Can you work these out from the model? Positions are in its coordinate system, mm. A direction names the side the tool comes from. Coordinates: 2 decimals unless noted, no trailing zeros. Order: outer loops, then holes, each group sorted by start corner. A loop starts at its lowest first (then second) coordinate and runs counter-clockwise, first axis right, second up. Notation, with made-up numbers: M -9.5,-7 L 36.5,-7 A26 ccw 36.5,29 Z; hole C -8.75,13 d3. An arc over 180 degrees is marked long. Answer as a JSON object with one key per item and string values.
from build123d import *

# Parameters (mm, degrees)
SKETCH1_W             = 28.575
SKETCH1_H             = 81.28
BOSS_EXTRUDE1_DEPTH   = 4.7625
SKETCH2_W             = 19.05
SKETCH2_H             = 25.4
CUT_EXTRUDE1_DEPTH    = 44.340785209
FILLET1_R             = 3.302
F_4_40_TAPPED_HOLE1_D = 2.2606


with BuildPart() as part:
    # Sketch1 → Boss-Extrude1 (new body)
    with BuildSketch(Plane.XY):
        Rectangle(SKETCH1_W, SKETCH1_H)
    extrude(amount=BOSS_EXTRUDE1_DEPTH)

    # Sketch2 → Cut-Extrude1 (cut, through all)
    with BuildSketch(Plane.XY.offset(4.7625)):
        with Locations((0, 17.78)):
            Rectangle(SKETCH2_W, SKETCH2_H)
        with Locations((0, -17.78)):
            Rectangle(SKETCH2_W, SKETCH2_H)
    extrude(amount=-CUT_EXTRUDE1_DEPTH, mode=Mode.SUBTRACT)

    # Fillet1
    fillet1_edges = [part.edges().sort_by_distance(p)[0] for p in [
        (9.525, 30.48, 2.38125),
        (9.525, 5.08, 2.38125),
        (-9.525, 5.08, 2.38125),
        (-9.525, 30.48, 2.38125),
        (-9.525, -30.48, 2.38125),
        (-9.525, -5.08, 2.38125),
        (9.525, -5.08, 2.38125),
        (9.525, -30.48, 2.38125),
    ]]
    fillet(fillet1_edges, radius=FILLET1_R)

    # #4-40 Tapped Hole1 (through all)
    with Locations(Plane(origin=(14.2875, 0, 0), x_dir=(0, 0, -1), z_dir=(1, 0, 0))):
        with Locations((-2.38125, 35.56), (-2.38125, 0), (-2.38125, -35.56)):
            Hole(F_4_40_TAPPED_HOLE1_D / 2)


solid = part.part
Item 1: I want a section at A-A, the plane x = -5.5. Write out the boundary of the cut face in (y, z).
Answers follow:
{"outline": "M -40.64,0 L -30.48,0 L -30.48,4.76 L -40.64,4.76 Z; M -5.08,0 L 5.08,0 L 5.08,4.76 L -5.08,4.76 Z; M 30.48,0 L 40.64,0 L 40.64,4.76 L 30.48,4.76 Z; hole C -35.56,2.38 d2.26; hole C 0,2.38 d2.26; hole C 35.56,2.38 d2.26"}
Item 2: Please list where these lines run through material, in increasing order: line 1 (Y direction, x = -6.5, z = 1); line 2 (X direction, y = -9, z = 0.4) (1 decimal); line 3 (Y direction, x = -6.25, z = 2.7).
Answers follow:
{"line 1": "y = -40.64 to -30.47, -5.09 to 5.09, 30.47 to 40.64", "line 2": "x = -14.3 to -9.5, 9.5 to 14.3", "line 3": "y = -40.64 to -36.64, -34.48 to -30.48, -5.08 to -1.08, 1.08 to 5.08, 30.48 to 34.48, 36.64 to 40.64"}
Item 3: I want a section at C-C, the plane y = -20. Write out the boundary of the cut face in (x, z) (1 decimal), plus the area to 3 significant figures.
Answers follow:
{"outline": "M -14.3,0 L -9.5,0 L -9.5,4.8 L -14.3,4.8 Z; M 9.5,0 L 14.3,0 L 14.3,4.8 L 9.5,4.8 Z", "area": "45.4 mm^2"}
Item 4: Which directions (+Z, -Z, +X, -X, +Y, -Y) give clear straight access to the entire face, cutting with the end or side of a thin tool? Please do faces 4 (the flat face through (0, 40.64, 2)), 5 (the cylindrical face through (-8.53, 29.54, 2.35)).
Answers follow:
{"face 4": "+Z, -Z, +X, -X, +Y", "face 5": "+Z, -Z"}
Item 5: I want a section at B-B, the plane y = 35.56. Write out the boundary of the cut face in (x, z), plus the area to 3 significant figures.
Answers follow:
{"outline": "M -14.29,0 L 14.29,0 L 14.29,1.25 L -14.29,1.25 Z; M -14.29,3.51 L 14.29,3.51 L 14.29,4.76 L -14.29,4.76 Z", "area": "71.5 mm^2"}
Item 6: If we mould it in two halves opening along Z, with no side actions, what happens to faces 1 (the flat face through (0, 1, 0)), 2 (the flat face through (0, 5.08, 2)), 3 (the cylindrical face through (-0.2, -34.44, 2.23))? For each: pulls with the +Z half, pulls with the -Z half, needs draft (parallel to the pull), parting line crosses it, or undercut.
Answers follow:
{"face 1": "pulls with the -Z half", "face 2": "needs draft", "face 3": "undercut"}
